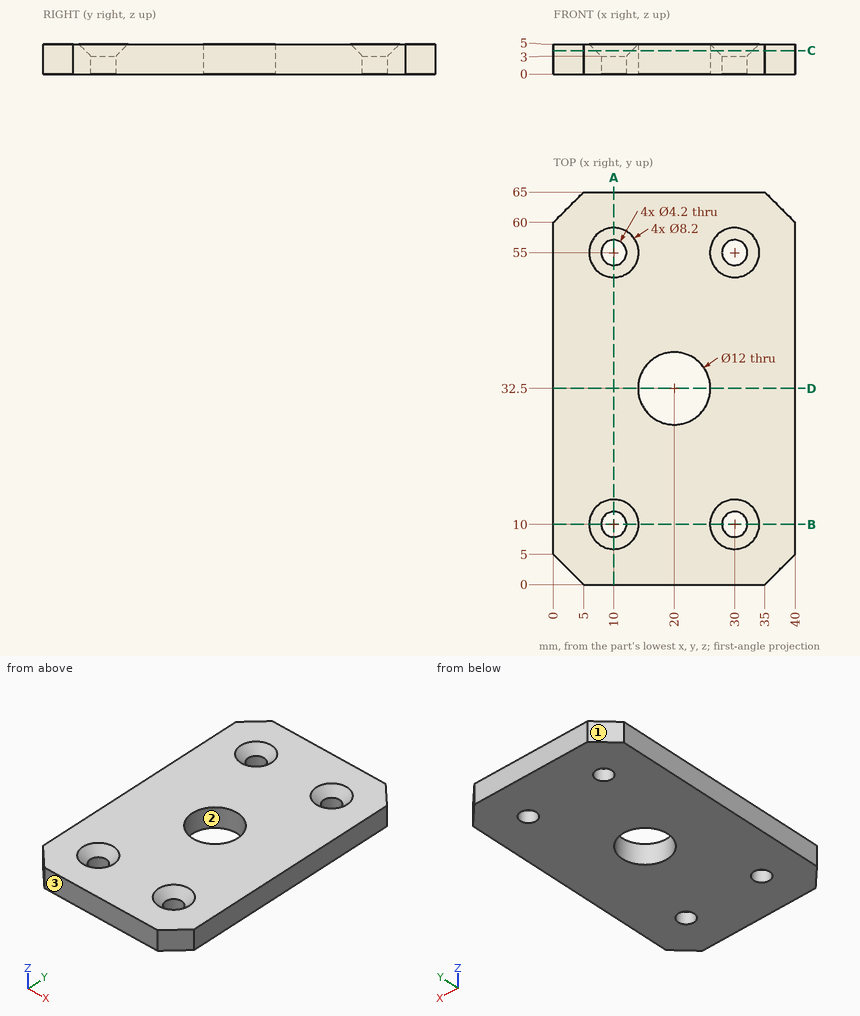
The figure shows three views and two pictorial views of one solid part (mm, origin at its lowest corner). Answer the questions. Give positions to 0.01 mm unless a question says otherwise; leave off trailing zeros. Write each loop counter-clockwise with the first axis right and the second up, starting at its lowest first coordinate (ties: lowest second). Pieces come first, ordered by that corner, then holes. Notation, with made-up numbers: M -24.75,-1 L -9.75,-1 A15 ccw -9.75,11 Z; hole C 41,-26 d8. An arc over 180 degrees is marked long. Write each question's results on one line, items separated by ' | '.
Q1. Section D-D, the plane y = 32.5 is taken. Write down the section's boundary in (x, z), then the cut area to 3 significant figures.
Output values:
outline: M 0,0 L 14,0 L 14,5 L 0,5 Z; M 26,0 L 40,0 L 40,5 L 26,5 Z | area: 140 mm2
Q2. Consider L1, parallel to Y at x = 30, z = 1.45; L2, parallel to X at y = 55, z = 2.35; L3, parallel to Y at x = 16, z = 0.9. Determine where each line is inside the solid, lowest interval first. Write a range as from..to.
Output values:
L1: 0..7.9, 12.1..52.9, 57.1..65 | L2: 0..7.9, 12.1..27.9, 32.1..40 | L3: 0..28.03, 36.97..65
Q3. For a pull along Y with two mould halves and no side action, classify the marked faces 1, 2 and 3 as released by +Y, released by -Y, zero draft, split by the parting line, or undercut.
Output values:
face 1: released by +Y | face 2: undercut | face 3: released by -Y
Q4. Section C-C, the plane z = 3.9 is taken. Write down the section's boundary in (x, y).
Output values:
outline: M 0,5 L 5,0 L 35,0 L 40,5 L 40,60 L 35,65 L 5,65 L 0,60 Z; hole C 10,10 d6; hole C 10,55 d6; hole C 20,32.5 d12; hole C 30,10 d6; hole C 30,55 d6
Q5. A flat-ended cylindrical pin translates along its axis: P1, Ø2, axis at x = 10, y = 52, coming from the +Z side. Find the tip coordinate at first contact, or state that the pin passes through.
Output values:
P1: z = 4.9
Q6. Section B-B, the plane y = 10 is taken. Write down the section's boundary in (x, z), then the cut area to 3 significant figures.
Output values:
outline: M 0,0 L 7.9,0 L 7.9,3 L 5.9,5 L 0,5 Z; M 12.1,0 L 27.9,0 L 27.9,3 L 25.9,5 L 14.1,5 L 12.1,3 Z; M 32.1,0 L 40,0 L 40,5 L 34.1,5 L 32.1,3 Z | area: 150 mm2
Q7. Section A-A, the plane x = 10 is taken. Write down the section's boundary in (y, z).
Output values:
outline: M 0,0 L 7.9,0 L 7.9,3 L 5.9,5 L 0,5 Z; M 12.1,0 L 52.9,0 L 52.9,3 L 50.9,5 L 14.1,5 L 12.1,3 Z; M 57.1,0 L 65,0 L 65,5 L 59.1,5 L 57.1,3 Z
